For this review, take the finished solid that the model builds, in its own axes (mm). A direction names the side the tool comes from. Give positions to 0.01 mm unless a question says otherwise; leave off trailing zeros. Order: outer loops, then holes, each group sorted by start corner. A loop starts at its lowest first (then second) coordinate and runs counter-clockwise, first axis right, second up. Notation, with made-up numbers: (-31, -12) - (21, -12) arc R31 cw to (21, 24) - close; hole circle Ø7 at (51.5, -15). An arc over 180 degrees is marked (long way). One line per item, written item: value.
Autodesk Inventor part; units mm, degrees
ref_plane "Start plane" through (0, 0, 0) normal (0, 0, 1) x (1, 0, 0)
ref_plane "End plane" through (0, 0, 609.6) normal (0, 0, 1) x (1, 0, 0)
ref_plane "YZ Plane" through (0, 0, 0) normal (1, 0, 0) x (0, 1, 0)
ref_plane "Start plane" through (0, 0, 0) normal (0, 0, 1) x (1, 0, 0)
ref_plane "End plane" through (0, 0, 609.6) normal (0, 0, 1) x (1, 0, 0)
sketch "Sketch" plane through (0, 0, 0) normal (0, 0, 1) x (1, 0, 0)
  line L0 (25.4, 0) -> (0, 0)
  line L1 (0, 0) -> (0, 25.4)
  line L2 (0, 25.4) -> (1.651, 25.4)
  line L3 (3.175, 23.876) -> (3.175, 6.477)
  line L4 (6.477, 3.175) -> (23.876, 3.175)
  line L5 (25.4, 1.651) -> (25.4, 0)
  line L6 (0, -11.0414) -> (0, 31.5385) construction
  line L7 (-11.0414, 0) -> (31.5385, 0) construction
  arc A0 (3.175, 6.477) -> (6.477, 3.175) centre (6.477, 6.477) ccw
  arc A1 (3.175, 23.876) -> (1.651, 25.4) centre (1.651, 23.876) ccw
  arc A2 (25.4, 1.651) -> (23.876, 3.175) centre (23.876, 1.651) ccw
  line L8 (0, 40.0545) -> (0, -19.5574) construction
  line L9 (-19.5574, 0) -> (40.0545, 0) construction
  point P0 (3.175, 25.4)
  point P1 (3.175, 3.175)
  point P2 (25.4, 3.175)
  dimension "d0" = 25.4
  dimension "d1" = 25.4
  dimension "d2" = 3.175
  dimension "d3" = 3.175
  dimension "d10" = 0
  dimension "d11" = 0
  dimension "d14" = 3.302
  dimension "d15" = 1.524
extrude "Body" add sketch "Sketch" along normal up to surface (609.6 mm away) from surface at 0
sketch "Sketch3" plane through (0, 0, 0) normal (0, 0, 1) x (1, 0, 0)
  line L0 (0, 0) -> (10, 0)
ref_plane "Work Plane3" through (0, 0, 0) normal (0, -1, 0) x (1, 0, 0)
sketch "Sketch4" plane through (0, 0, 0) normal (0, -1, 0) x (1, 0, 0)
  line L0 (-2, 0) -> (12, 0)
  line L1 (-2, 609.6) -> (12, 609.6)
  dimension "d17" = 609.6
sketch "Sketch6" plane through (0, 0, 0) normal (0, -1, 0) x (1, 0, 0)
  line L0 (25.4, 590.55) -> (12.7, 590.55)
  line L1 (12.7, 580.55) -> (25.4, 580.55)
  line L2 (25.4, 580.55) -> (25.4, 590.55)
  arc A0 (12.7, 590.55) -> (12.7, 580.55) centre (15.8943, 585.55) ccw
  line L3 (25.4, 609.6) -> (0, 609.6)
  line L4 (25.4, 0) -> (25.4, 609.6)
  point P0 (0, 0)
  dimension "d23" = 12.7
  dimension "d24" = 10
  dimension "d28" = 19.05
extrude "Extrusion3" cut sketch "Sketch6" against normal up to surface (3.175 mm away)
equation "\"d0\" = G_H"
equation "\"d1\" = G_H"
equation "\"d2\" = G_T"
equation "\"d3\" = G_T"
equation "\"d14\" = G_IR"
equation "\"d15\" = G_ER"
equation "\"d4\" = G_L"
equation "\"d23\" = axle_inset_up"
equation "\"d28\" = axle_inset_fwd"
equation "\"G_H\" = 25.4"
equation "\"G_T\" = 3.175"
equation "\"G_ER\" = 1.524"
equation "\"G_IR\" = 3.302"
equation "\"G_L\" = d17"
equation "\"ex\" = 0"
equation "\"G_OFFSET_START\" = 0"
equation "\"G_OFFSET_END\" = 0"
equation "\"d13\" = G_OFFSET_END + B_L"
equation "\"B_L\" = 609.6"
equation "\"axle_inset_fwd\" = 19.05"
equation "\"axle_inset_up\" = 12.7"
properties part number "AISC - L 1 x 1 x 1/8 - 24" material "Steel, Mild"
(1) Wall thickness on line 1 (Y direction, x = 21.75, z = 115) (3 decimals); line 2 (Z direction, x = 18.5, y = 1.5): over which ranges is each line inside the solid? List them lowest first. Write a range as from..to.
Answers below:
line 1: y = 0..3.175
line 2: z = 0..580.55, 590.55..609.6
(2) Machinability: for faces 1 (the face through (3.175, 15, 301)), 2 (the face through (3, 5, 609.6)), which of the approach directions +Z, -Z, +X, -X, +Y, -Y give a long, thin tool a straight path to every point of the face, cutting with its end or side? Answer none if there is none.
Answers below:
face 1: +Z, -Z, +X, +Y
face 2: +Z, +X, -X, +Y, -Y
(3) Take a section at C-C (y = 19.75). Write out the cut boundary in (x, z) (3 decimals), then the cut area to 3 significant figures.
Answers below:
outline: (0, 0) - (3.175, 0) - (3.175, 609.6) - (0, 609.6) - close
area: 1,940 mm^2
(4) Take a section at B-B (z = 221). Write out the cut boundary in (x, y) (3 decimals), then the cut area to 3 significant figures.
Answers below:
outline: (0, 0) - (25.4, 0) - (25.4, 1.651) arc R1.524 ccw to (23.876, 3.175) - (6.477, 3.175) arc R3.302 cw to (3.175, 6.477) - (3.175, 23.876) arc R1.524 ccw to (1.651, 25.4) - (0, 25.4) - close
area: 153 mm^2
(5) Take a section at A-A (x = 18.75). Write out the cut boundary in (y, z) (3 decimals).
Answers below:
outline: (0, 0) - (3.175, 0) - (3.175, 580.55) - (0, 580.55) - close; (0, 590.55) - (3.175, 590.55) - (3.175, 609.6) - (0, 609.6) - close
(6) For P1, Ø4, axis at y = 22, z = 275, coming from the +X side (3 decimals); P2, Ø10, axis at y = 8, z = 252.5, coming from the +X side; P3, Ø2, axis at x = 9, z = 276, coming from the +Y side (3 decimals), all flat-tipped, find the tip position at first contact; note any pin that passes through.
Answers below:
P1: stops at x = 3.175
P2: stops at x = 24.59
P3: stops at y = 3.175
